Geometry: final body of the model. Coordinates: model frame, mm. A direction names the side the tool comes from. Coordinates: 2 decimals unless noted, no trailing zeros. Loops run counter-clockwise (first coordinate to the right, second up) from the corner with the lowest first, then second, coordinate; pieces in that order, holes last. Notation, with made-up numbers: M -30.5,6 L -10.5,6 A34 cw -10.5,45 Z; hole C -10.75,9.25 d1. An arc over 180 degrees is marked long. Write each question's results on one line, items separated by ' | '. Start each with the question number.
from build123d import *

# Parameters (mm, degrees)
F0_R     = 2
F1_DEPTH = 2
F3_DEPTH = 30


# Not quite as in the source:
# - ends of sketch curves that miss each other by under 0.0002 mm in the source are joined
# - a feature names something its author has since deleted; it is built from what else it names


with BuildPart() as f1:
    # F0 (on Right) → F1 (new body)
    with BuildSketch(Plane.YZ):
        with BuildLine():
            Line((-34.5930008724, 26.4829086736), (-38.1068567038, 26.4829086736))
            Line((-38.1068567038, 26.4829086736), (-38.1068567038, -3.5426183596))
            Line((-38.1068567038, -3.5426183596), (-34.5929991737, -3.5426183596))
            Line((-34.5929991737, -3.5426183596), (-34.5929991737, -1.9446051591))
            ThreePointArc((-34.5929991737, -1.9446051591), (-34.2912179318, -0.233833257), (-33.4223029733, 1.2704270974))
            Line((-33.4223029733, 1.2704270974), (-31.3919489583, 3.6887052743))
            Line((-31.3919489583, 3.6887052743), (-30.7011796085, 4.5114546232))
            ThreePointArc((-30.7011796085, 4.5114546232), (-28.9149664525, 5.8599495795), (-26.7193999751, 6.2940969379))
            ThreePointArc((-26.7193999751, 6.2940969379), (-22.9223984991, 9.7713294978), (-26.2963942816, 13.660354947))
            ThreePointArc((-26.2963942816, 13.660354947), (-28.3284558204, 14.2855279257), (-29.9170611144, 15.6984853104))
            Line((-29.9170611144, 15.6984853104), (-33.634288291, 20.8009439295))
            ThreePointArc((-33.634288291, 20.8009439295), (-34.3472851032, 22.1969357772), (-34.5930008724, 23.7450899858))
            Line((-34.5930008724, 23.7450899858), (-34.5930008724, 26.4829086736))
        make_face()
        with BuildLine():
            ThreePointArc((-29.6578618205, 11.6234470561), (-29.4825953492, 11.2153956919), (-29.5013036541, 10.771690552))
            ThreePointArc((-29.5013036541, 10.771690552), (-29.6050814327, 10.0861001216), (-29.5486860291, 9.3949969281))
            ThreePointArc((-29.5486860291, 9.3949969281), (-29.5605283151, 8.9510554769), (-29.7634350443, 8.5560198949))
            Line((-29.7634350443, 8.5560198949), (-33.8409951472, 3.699391672))
            ThreePointArc((-33.8409951472, 3.699391672), (-34.9490102875, 3.4027543717), (-35.6068559071, 4.3423981233))
            Line((-35.6068559071, 4.3423981233), (-35.6068559071, 16.7184074453))
            ThreePointArc((-35.6068559071, 16.7184074453), (-34.9164867488, 17.6692642914), (-33.7985984234, 17.3072366565))
            Line((-33.7985984234, 17.3072366565), (-29.6578618205, 11.6234470561))
        make_face(mode=Mode.SUBTRACT)
        with Locations((-26.6068567038, 9.9829086736)):
            Circle(F0_R, mode=Mode.SUBTRACT)
    extrude(amount=F1_DEPTH)

    # F2 (on face) → F3 (join)
    with BuildSketch(Plane(origin=(0, 0, -3.5426183596), x_dir=(1, 0, 0), z_dir=(0, 0, -1))):
        with BuildLine():
            Line((-1.0014715791, 45.0346349695), (2.9985283307, 45.035484586))
            Line((2.9985283307, 45.035484586), (4.9992640751, 41.5718078573))
            Line((4.9992640751, 41.5718078573), (2.9999999098, 38.107281512))
            Line((2.9999999098, 38.107281512), (0.9999999926, 38.1068567038))
            Line((0.9999999926, 38.1068567038), (2, 38.1068567038))
            Line((2, 38.1068567038), (2, 36.6721290144))
            ThreePointArc((2, 36.6721290144), (4.8724849939, 38.4089714581), (5.9992641654, 41.5709582407))
            ThreePointArc((5.9992641654, 41.5709582407), (-2.1633043456, 45.4437040901), (0, 36.6718286111))
            Line((0, 36.6718286111), (0, 38.1066442996))
            Line((0, 38.1066442996), (-1, 38.1064318955))
            Line((-1, 38.1064318955), (-3.0007357444, 41.5701086242))
            Line((-3.0007357444, 41.5701086242), (-1.0014715791, 45.0346349695))
        make_face()
    extrude(amount=-F3_DEPTH)


solid = f1.part
Item 1: Contact query for flat-ended pins moving along their axis: P1, Ø3, axis at x = 0.5, y = -32, coming from the -Z side; P2, Ø4.5, axis at y = -30.5, z = 18, coming from the -X side; P3, Ø1.5, axis at y = -30.5, z = 5, coming from the +X side. Output: stop coordinate, or through.
Item 2: Section A-A, the plane y = -44.25. Return loops of the section in (x, z).
Item 3: Ray query, L1, parallel to Y at x = 1.5, z = 16; L2, parallel to Z at x = 2.25, y = -45.5; L3, parallel to X at y = -44.75, z = 1.5. Return the intervals inside material, ascending. Write a range as [from, to].
Item 4: Pull-direction query (Y, two-part tool) for faces 5 (the flat face through (1, -34.593, -3)), 6 (the flat face through (0.99, -31.76, 14.51)), 7 (the flat face through (1, -37.9, -3.543)); classes: released by +Y, released by -Y, zero draft, split by the parting line, or undercut.
Item 5: Section C-C, the plane x = -1.5. Return loops of the section in (y, z), plus the area to 3 significant figures.
Item 6: Set-up query: faces 1 (the flat face through (1, -34.593, 25)), 2 (the flat face through (1, -36, 26.483)), 3 (the flat face through (4, -43.3, 11.2)), 4 (the cylindrical face through (0.986, -34.933, 3.397)). Return all of +Z, -Z, +X, -X, +Y, -Y with unobstructed straight access to the full face (end or side cutting, diameter ignored); none if empty.
Item 7: Section B-B, the plane z = 7. Count the separate pieces of the cut face and the enclosed holes in it, plus the area to 3 significant figures.
Solutions:
1) P1: stops at z = 1.18 | P2: stops at x = 0 | P3: stops at x = 2
2) outline: M -3.22,-3.54 L -1.45,-3.54 L -1.45,26.46 L -3.22,26.46 Z; M 3.45,-3.54 L 5.22,-3.54 L 5.22,26.46 L 3.45,26.46 Z
3) L1: y = [-46.55, -45.04], [-38.11, -35.61], [-32.85, -30.14] | L2: z = [-3.54, 26.46] | L3: x = [-2.86, -1.17], [3.16, 4.86]
4) face 5: released by +Y | face 6: undercut | face 7: zero draft
5) outline: M -45.9,-3.54 L -44.17,-3.54 L -44.17,26.46 L -45.9,26.46 Z; M -38.97,-3.54 L -37.24,-3.54 L -37.24,26.46 L -38.97,26.46 Z | area: 104 mm²
6) face 1: +Z, +X, -X, +Y | face 2: +Z, +X, -X, +Y, -Y | face 3: +Z, -Z | face 4: +X, -X
7) separate pieces: 2 | enclosed holes: 1 | area: 52.2 mm²
